Geometry check sheet. Reference: drawing and pictorial views, mm from the part's lowest x, y, z. A direction names the side the tool comes from. Round coordinates to 2 decimals unless told otherwise and drop trailing zeros. Loops run counter-clockwise (first coordinate to the right, second up) from the corner with the lowest first, then second, coordinate; pieces in that order, holes last. Notation, with made-up numbers: (84.25, -3.75) -> (116.25, -3.75) arc R26 ccw to (116.25, 12.25) -> close; hole circle Ø3 at (32, 72). An arc over 180 degrees is marked (long way). Use one line per item in the form item = value.
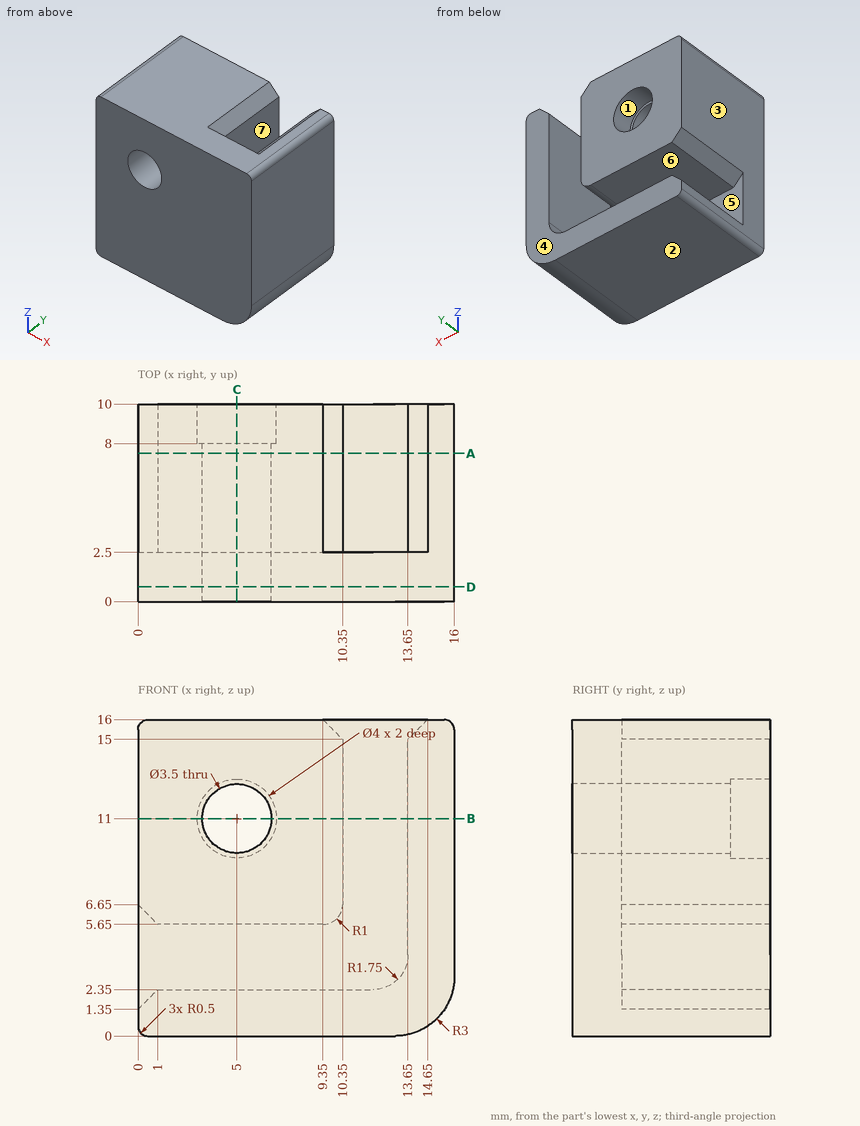
1. Section check D-D (y = 0.75). Record the boundary of the cut face in (x, z), then the cut area to 3 significant figures.
Return value:
outline = (0, 0.5) arc R0.5 ccw to (0.5, 0) -> (13, 0) arc R3 ccw to (16, 3) -> (16, 15.5) arc R0.5 ccw to (15.5, 16) -> (0.5, 16) arc R0.5 ccw to (0, 15.5) -> close; hole circle Ø3.5 at (5, 11)
area = 244 mm2
2. Section check C-C (x = 5). Record the boundary of the cut face in (y, z), then the cut area to 4 significant figures.
Return value:
outline = (0, 0) -> (10, 0) -> (10, 2.35) -> (2.5, 2.35) -> (2.5, 5.65) -> (10, 5.65) -> (10, 9) -> (8, 9) -> (8, 9.25) -> (0, 9.25) -> close; (0, 12.75) -> (8, 12.75) -> (8, 13) -> (10, 13) -> (10, 16) -> (0, 16) -> close
area = 99.25 mm2
3. Material ranges on line 1 along X through (y, z) = (8.8, 11); line 2 along X through (y, z) = (3.5, 11); line 3 along X through (y, z) = (8.5, 14), recorded low to high.
Return value:
line_1 = 0 to 3, 7 to 10.35, 13.65 to 16
line_2 = 0 to 3.25, 6.75 to 10.35, 13.65 to 16
line_3 = 0 to 10.35, 13.65 to 16
4. Section check B-B (z = 11). Record the boundary of the cut face in (x, y), then the cut area to 4 significant figures.
Return value:
outline = (0, 0) -> (3.25, 0) -> (3.25, 8) -> (3, 8) -> (3, 10) -> (0, 10) -> close; (6.75, 0) -> (16, 0) -> (16, 10) -> (13.65, 10) -> (13.65, 2.5) -> (10.35, 2.5) -> (10.35, 10) -> (7, 10) -> (7, 8) -> (6.75, 8) -> close
area = 99.25 mm2
5. Section check A-A (y = 7.5). Record the boundary of the cut face in (x, z).
Return value:
outline = (0, 0.5) arc R0.5 ccw to (0.5, 0) -> (13, 0) arc R3 ccw to (16, 3) -> (16, 15.5) arc R0.5 ccw to (15.5, 16) -> (14.65, 16) -> (13.65, 15) -> (13.65, 4.1) arc R1.75 cw to (11.9, 2.35) -> (1, 2.35) -> (0, 1.35) -> close; (0, 6.65) -> (1, 5.65) -> (9.35, 5.65) arc R1 ccw to (10.35, 6.65) -> (10.35, 15) -> (9.35, 16) -> (0.5, 16) arc R0.5 ccw to (0, 15.5) -> close; hole circle Ø3.5 at (5, 11)
6. Gauge pin test, flat end, axial feed: pin 1 (2 mm diameter, centred on x = 4, z = 11.5, fed in from +Y). Record the tip position at first contact, or that the pin passes through.
Return value:
pin_1 = 10
7. Mould release check, pull along Z, two halves, no side actions. Record for the marked faces 1, 2 and 3: released by +Z, released by -Z, zero draft, split by the parting line, or undercut.
Return value:
face_1 = undercut
face_2 = released by -Z
face_3 = zero draft
8. Tool access check on the marked faces 4, 5, 6 and 7. Record the directions out of +Z, -Z, +X, -X, +Y, -Y that give a thin tool (end or side, any length) a straight path to the whole face; none if there is none.
Return value:
face_4 = +Z, -Z, +X, -X, +Y
face_5 = +Y
face_6 = -X, +Y
face_7 = +Z, +Y
